Check sheet for the modelled part. Datum: model origin and axes. Units: mm. Face numbers are marked on the shaded views. A direction names the side the tool comes from. Give positions to 0.01 mm unless a question says otherwise; leave off trailing zeros. Loops run counter-clockwise (first coordinate to the right, second up) from the corner with the lowest first, then second, coordinate; pieces in that order, holes last. Notation, with made-up numbers: (-33.75, 64) -> (-0.75, 64) arc R19 cw to (-0.75, 87) -> close; hole circle Ø4 at (-27.5, 44). An arc over 180 degrees is marked (long way). Write each question's results on one line, items separated by ' | '. Start each with the question number.
1. Cross-section at A-A on y = 145. Record the boundary of the cut face in (x, z).
2. Gauge pin test, flat ends, axial feed: pin 1 Ø8 at (x, z) = (-90, -15) entering from +Y; pin 2 Ø4 at (x, z) = (78.5, -27) entering from -Y; pin 3 Ø10 at (x, y) = (79, 82.5) entering from -Z. Record the tip position at first contact, or that the pin passes through.
3. Mould release check, pull along Y, two halves, no side actions. Record for the marked faces 1, 2, 3 and 4: +Y half, -Y half, draft (parallel to the pull), parting line (faces both ways), or undercut.
4. Cross-section at B-B on z = 0. Record the boundary of the cut face in (x, y), and give its area (3 significant figures).
5. Material ranges on L1, parallel to Y at x = 0, z = -47.75; L2, parallel to Y at x = 0, z = 54; L3, parallel to Z at x = -36.5, y = 127.5, recorded low to high. Write a range as from..to.
6. Cross-section at C-C on x = -34. Record the boundary of the cut face in (y, z).
7. Tool access check on the marked faces 5, 6 and 7. Record the directions out of +Z, -Z, +X, -X, +Y, -Y that give a thin tool (end or side, any length) a straight path to the whole face; none if there is none.
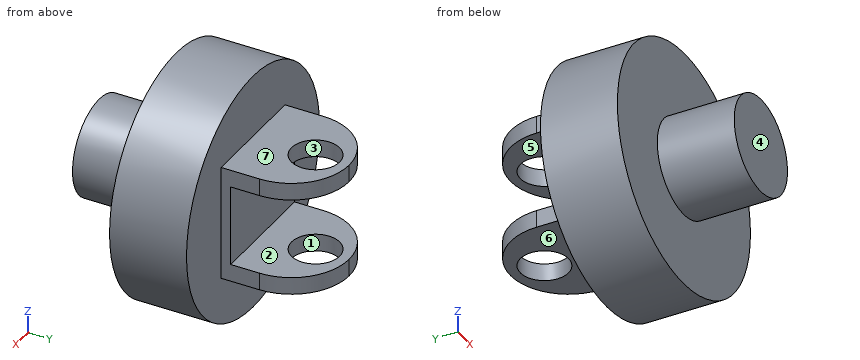
from build123d import *

# Parameters (mm, degrees)
SKETCH1_R           = 125
BOSS_EXTRUDE1_DEPTH = 80
SKETCH2_R           = 50
BOSS_EXTRUDE2_DEPTH = 160
SKETCH3_W           = 120
SKETCH3_H           = 120
BOSS_EXTRUDE3_DEPTH = 100
SKETCH4_W           = 120
SKETCH4_H           = 84
CUT_EXTRUDE1_DEPTH  = 90
FILLET1_R           = 60
SKETCH5_R           = 25
CUT_EXTRUDE2_DEPTH  = 130


with BuildPart() as part:
    # Sketch1 → Boss-Extrude1 (new body)
    with BuildSketch(Plane(origin=(0, 0, 0), x_dir=(1, 0, 0), z_dir=(0, 1, 0))):
        with Locations(Location((0, 0, 0), (0, 0, 270))):
            Circle(SKETCH1_R)
    extrude(amount=BOSS_EXTRUDE1_DEPTH)

    # Sketch2 → Boss-Extrude2 (add)
    with BuildSketch(Plane(origin=(0, 80, 0), x_dir=(1, 0, 0), z_dir=(0, 1, 0))):
        with Locations(Location((0, 0, 0), (0, 0, 270))):
            Circle(SKETCH2_R)
    extrude(amount=-BOSS_EXTRUDE2_DEPTH)

    # Sketch3 → Boss-Extrude3 (add)
    with BuildSketch(Plane(origin=(0, 80, 0), x_dir=(1, 0, 0), z_dir=(0, 1, 0))):
        Rectangle(SKETCH3_W, SKETCH3_H)
    extrude(amount=BOSS_EXTRUDE3_DEPTH)

    # Sketch4 → Cut-Extrude1 (cut)
    with BuildSketch(Plane(origin=(0, 180, 0), x_dir=(1, 0, 0), z_dir=(0, 1, 0))):
        Rectangle(SKETCH4_W, SKETCH4_H)
    extrude(amount=-CUT_EXTRUDE1_DEPTH, mode=Mode.SUBTRACT)

    # Fillet1
    fillet1_edges = [part.edges().sort_by_distance(p)[0] for p in [
        (-60, 180, 51),
        (-60, 180, -51),
        (60, 180, -51),
        (60, 180, 51),
    ]]
    fillet(fillet1_edges, radius=FILLET1_R - 0.0001)  # a hair under: the kernel refuses the full size

    # Sketch5 → Cut-Extrude2 (cut)
    with BuildSketch(Plane.XY.offset(60)):
        with Locations((0, 145)):
            Circle(SKETCH5_R)
    extrude(amount=-CUT_EXTRUDE2_DEPTH, mode=Mode.SUBTRACT)


solid = part.part
Geometry says:
1) outline: (-54.54, -60) -> (-25, -60) -> (-25, -42) -> (-54.54, -42) -> close; (-54.54, 42) -> (-25, 42) -> (-25, 60) -> (-54.54, 60) -> close; (25, -60) -> (54.54, -60) -> (54.54, -42) -> (25, -42) -> close; (25, 42) -> (54.54, 42) -> (54.54, 60) -> (25, 60) -> close
2) pin 1: y = 80 | pin 2: y = 0 | pin 3: z = -100.25
3) face 1: undercut | face 2: draft | face 3: undercut | face 4: -Y half
4) outline: (-125, 0) -> (-50, 0) -> (-50, -80) -> (50, -80) -> (50, 0) -> (125, 0) -> (125, 80) -> (60, 80) -> (60, 90) -> (-60, 90) -> (-60, 80) -> (-125, 80) -> close | area: 29,200 mm^2
5) L1: -80..120, 170..180 | L2: 0..120, 170..180 | L3: -60..-42, 42..60
6) outline: (-80, -36.66) -> (0, -36.66) -> (0, -120.29) -> (80, -120.29) -> (80, -60) -> (169.44, -60) -> (169.44, -42) -> (90, -42) -> (90, 42) -> (169.44, 42) -> (169.44, 60) -> (80, 60) -> (80, 120.29) -> (0, 120.29) -> (0, 36.66) -> (-80, 36.66) -> close
7) face 5: +X, -X, +Y | face 6: -Z, +X, -X, +Y | face 7: +Z, +X, -X, +Y
